Design review of the part built by this model. Coordinates are the model's own, in mm. Face numbers are marked on the shaded views. A direction names the side the tool comes from. Coordinates: 2 decimals unless noted, no trailing zeros. Loops run counter-clockwise (first coordinate to the right, second up) from the corner with the lowest first, then second, coordinate; pieces in that order, holes last. Notation, with made-up numbers: M -23,74.5 L -8,74.5 A31 cw -8,111.5 Z; hole C 26.25,76.25 d11. An arc over 180 degrees is marked long. Write item = value, one per line. Start each with the question number.
Autodesk Inventor part; units mm, degrees
ref_plane "YZ Plane" through (0, 0, 0) normal (1, 0, 0) x (0, 1, 0)
ref_plane "XZ Plane" through (0, 0, 0) normal (0, 1, 0) x (-1, 0, 0)
ref_plane "XY Plane" through (0, 0, 0) normal (0, 0, 1) x (1, 0, 0)
sketch "Boceto1" plane through (0, 0, 0) normal (0, 1, 0) x (-1, 0, 0)
  line L0 (200, 200) -> (-200, 200)
  line L1 (-200, 200) -> (-200, -200)
  line L2 (-200, -200) -> (200, -200)
  line L3 (200, -200) -> (200, 200)
  line L4 (195, 195) -> (-195, 195)
  line L5 (-195, 195) -> (-195, -195)
  line L6 (-195, -195) -> (195, -195)
  line L7 (195, -195) -> (195, 195)
  point P0 (0, 0)
  dimension "L" = 400
  dimension "d1" = 400
  dimension "d2" = 200
  dimension "d3" = 200
  dimension "d4" = 390
  dimension "d5" = 390
  dimension "d6" = 195
  dimension "d7" = 195
extrude "Extrusión1" add sketch "Boceto1" along normal blind 200
sketch "Boceto2" plane through (0, 0, 0) normal (0, -1, 0) x (1, 0, 0)
  line L0 (195, 195) -> (-195, 195)
  line L1 (-195, -195) -> (195, -195)
  line L2 (195, 195) -> (-195, 195)
  line L3 (-195, 195) -> (-195, -195)
  line L4 (-195, -195) -> (195, -195)
  line L5 (195, -195) -> (195, 195)
  point P0 (0, 0)
  point P1 (195, -195)
extrude "Extrusión2" add sketch "Boceto2" against normal blind 5
equation "\"d1\" = L"
properties part number "techo"
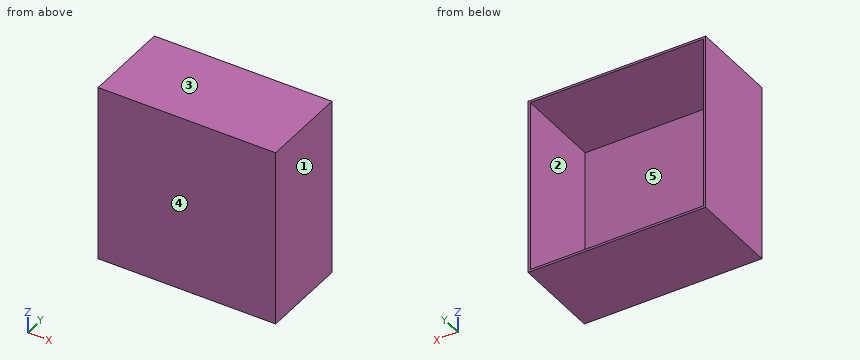
(1) To check wall thickness, follow L1, parallel to Z at x = 138, y = 169; L2, parallel to Y at x = 84.5, z = -155. State the ranges of each line that lie inside material, in increasing order.
(2) Take a section at B-B (x = 58). State the section outline as (y, z) points, plus the area to 3 significant figures.
(3) Tool access review of the marked faces 4 and 5: name each direction out of +Z, -Z, +X, -X, +Y, -Y from which nothing blocks a thin tool from reaching the whole face with its end or side.
(4) Take a section at A-A (y = 134). State the section outline as (x, z) points.
(5) Insertion check: pin 1 (12 mm diameter, centred on x = 130, z = -63, fed in from +Y). The pin has a flat end and moves straight along its axis. Give the tip position at first contact, or say it passes through.
(6) Take a section at C-C (z = -167). State the section outline as (x, y) points, plus the area to 3 significant figures.
(7) Mouldability with a two-part tool opening along Z and no side actions: class the marked faces 1, 2 and 3 as +Z half, -Z half, draft (parallel to the pull), parting line (faces both ways), or undercut.
Results list:
q1.L1 = -200 to -195, 195 to 200
q1.L2 = 0 to 5
q2.outline = M 0,-200 L 200,-200 L 200,-195 L 5,-195 L 5,195 L 200,195 L 200,200 L 0,200 Z
q2.area = 3,950 mm^2
q3.face_4 = +Z, -Z, +X, -X, -Y
q3.face_5 = +Y
q4.outline = M -200,-200 L 200,-200 L 200,200 L -200,200 Z; hole M -195,-195 L 195,-195 L 195,195 L -195,195 Z
q5.pin_1 = 5
q6.outline = M -200,0 L 200,0 L 200,200 L 195,200 L 195,5 L -195,5 L -195,200 L -200,200 Z
q6.area = 3,950 mm^2
q7.face_1 = draft
q7.face_2 = undercut
q7.face_3 = +Z half
